Autodesk Inventor part; units mm, degrees
ref_plane "YZ Plane" through (0, 0, 0) normal (1, 0, 0) x (0, 1, 0)
ref_plane "XZ Plane" through (0, 0, 0) normal (0, 1, 0) x (-1, 0, 0)
ref_plane "XY Plane" through (0, 0, 0) normal (0, 0, 1) x (1, 0, 0)
sketch "Sketch1" plane through (0, 0, 0) normal (0, 1, 0) x (-1, 0, 0)
  circle A0 centre (0, 0) radius 103.75 construction
  line L0 (0, -103.75) -> (-30, -103.75) construction
  line L1 (-30, -103.75) -> (-30, -99.318) construction
  line L2 (0, -103.75) -> (0, -91.6543) construction
  line L3 (0, 0) -> (-10.2863, 0) construction
  circle A1 centre (-30, -99.318) radius 1.6
  circle A2 centre (30, -99.318) radius 1.6
  circle A3 centre (-99.318, -30) radius 1.6
  circle A4 centre (-99.318, 30) radius 1.6
  arc A5 (53.1423, -96.3114) -> (51.7739, -97.0539) centre (0, 0) ccw construction
  arc A6 (43.0581, -98.5) -> (-43.0581, -98.5) centre (0, 0) ccw
  line L4 (0, -107.5) -> (0, -98.5) construction
  line L5 (0, -98.5) -> (0, -73.5) construction
  line L6 (0, -98.5) -> (-43.0581, -98.5) construction
  line L7 (0, -98.5) -> (43.0581, -98.5) construction
  line L8 (43.0581, -98.5) -> (-43.0581, -98.5) construction
  line L9 (-18.0581, -73.5) -> (18.0581, -73.5)
  arc A7 (43.0581, -98.5) -> (18.0581, -73.5) centre (18.0581, -98.5) ccw
  arc A8 (-18.0581, -73.5) -> (-43.0581, -98.5) centre (-18.0581, -98.5) ccw
  line L10 (0, 107.5) -> (0, 97.5) construction
  line L11 (0, 97.5) -> (-22.5, 97.5) construction
  line L12 (-22.5, 97.5) -> (-22.5, 82.5) construction
  line L13 (22.5, 82.5) -> (22.5, 97.5) construction
  line L14 (22.5, 90) -> (-22.5, 90) construction
  line L15 (15, 97.5) -> (-15, 97.5)
  line L16 (-15, 82.5) -> (15, 82.5)
  arc A9 (15, 82.5) -> (15, 97.5) centre (15, 90) ccw
  arc A10 (-15, 97.5) -> (-15, 82.5) centre (-15, 90) ccw
  line L17 (22.5, 82.5) -> (17.5, 82.5) construction
  line L18 (17.5, 82.5) -> (17.5, 77.5) construction
  circle A11 centre (17.5, 77.5) radius 1.6
  circle A12 centre (-17.5, 77.5) radius 1.6
  line L19 (-58.3363, 79.5495) -> (-79.5495, 58.3363)
  arc A13 (-47.7297, 68.9429) -> (-58.3363, 79.5495) centre (-53.033, 74.2462) ccw
  arc A14 (-79.5495, 58.3363) -> (-68.9429, 47.7297) centre (-74.2462, 53.033) ccw
  line L20 (-68.9429, 47.7297) -> (-47.7297, 68.9429)
  circle A15 centre (-67.1751, 42.4264) radius 1.6
  circle A16 centre (-42.4264, 67.1751) radius 1.6
  line L21 (-97.5, 15) -> (-97.5, -15)
  arc A17 (-82.5, 15) -> (-97.5, 15) centre (-90, 15) ccw
  arc A18 (-97.5, -15) -> (-82.5, -15) centre (-90, -15) ccw
  line L22 (-82.5, -15) -> (-82.5, 15)
  circle A19 centre (-77.5, -17.5) radius 1.6
  circle A20 centre (-77.5, 17.5) radius 1.6
  line L23 (-79.5495, -58.3363) -> (-58.3363, -79.5495)
  arc A21 (-68.9429, -47.7297) -> (-79.5495, -58.3363) centre (-74.2462, -53.033) ccw
  arc A22 (-58.3363, -79.5495) -> (-47.7297, -68.9429) centre (-53.033, -74.2462) ccw
  line L24 (-47.7297, -68.9429) -> (-68.9429, -47.7297)
  circle A23 centre (-42.4264, -67.1751) radius 1.6
  circle A24 centre (-67.1751, -42.4264) radius 1.6
  line L25 (-15, -97.5) -> (15, -97.5)
  arc A25 (-15, -82.5) -> (-15, -97.5) centre (-15, -90) ccw
  arc A26 (15, -97.5) -> (15, -82.5) centre (15, -90) ccw
  line L26 (15, -82.5) -> (-15, -82.5)
  circle A27 centre (17.5, -77.5) radius 1.6
  circle A28 centre (-17.5, -77.5) radius 1.6
  line L27 (58.3363, -79.5495) -> (79.5495, -58.3363)
  arc A29 (47.7297, -68.9429) -> (58.3363, -79.5495) centre (53.033, -74.2462) ccw
  arc A30 (79.5495, -58.3363) -> (68.9429, -47.7297) centre (74.2462, -53.033) ccw
  line L28 (68.9429, -47.7297) -> (47.7297, -68.9429)
  circle A31 centre (67.1751, -42.4264) radius 1.6
  circle A32 centre (42.4264, -67.1751) radius 1.6
  line L29 (97.5, -15) -> (97.5, 15)
  arc A33 (82.5, -15) -> (97.5, -15) centre (90, -15) ccw
  arc A34 (97.5, 15) -> (82.5, 15) centre (90, 15) ccw
  line L30 (82.5, 15) -> (82.5, -15)
  circle A35 centre (77.5, 17.5) radius 1.6
  circle A36 centre (77.5, -17.5) radius 1.6
  line L31 (79.5495, 58.3363) -> (58.3363, 79.5495)
  arc A37 (68.9429, 47.7297) -> (79.5495, 58.3363) centre (74.2462, 53.033) ccw
  arc A38 (58.3363, 79.5495) -> (47.7297, 68.9429) centre (53.033, 74.2462) ccw
  line L32 (47.7297, 68.9429) -> (68.9429, 47.7297)
  circle A39 centre (42.4264, 67.1751) radius 1.6
  circle A40 centre (67.1751, 42.4264) radius 1.6
  line L33 (58.3363, -58.3363) -> (51.2652, -51.2652) construction
  line L34 (40.6586, -61.8718) -> (61.8718, -40.6586)
  arc A41 (40.6586, -61.8718) -> (44.5267, -89.5398) centre (53.033, -74.2462) ccw
  arc A42 (89.5398, -44.5267) -> (61.8718, -40.6586) centre (74.2462, -53.033) ccw
  line L35 (0, -73.5) -> (0, -66.5) construction
  arc A43 (44.5267, 89.5398) -> (40.6586, 61.8718) centre (53.033, 74.2462) ccw
  line L36 (61.8718, 40.6586) -> (40.6586, 61.8718)
  arc A44 (61.8718, 40.6586) -> (89.5398, 44.5267) centre (74.2462, 53.033) ccw
  arc A45 (-89.5398, 44.5267) -> (-61.8718, 40.6586) centre (-74.2462, 53.033) ccw
  line L37 (-40.6586, 61.8718) -> (-61.8718, 40.6586)
  arc A46 (-40.6586, 61.8718) -> (-44.5267, 89.5398) centre (-53.033, 74.2462) ccw
  arc A47 (-44.5267, -89.5398) -> (-40.6586, -61.8718) centre (-53.033, -74.2462) ccw
  line L38 (-61.8718, -40.6586) -> (-40.6586, -61.8718)
  arc A48 (-61.8718, -40.6586) -> (-89.5398, -44.5267) centre (-74.2462, -53.033) ccw
  arc A49 (89.5398, -44.5267) -> (89.5398, 44.5267) centre (0, 0) ccw
  arc A50 (-89.5398, 44.5267) -> (-89.5398, -44.5267) centre (0, 0) ccw
  line L39 (43.0581, -98.5) -> (48.0581, -98.5) construction
  line L40 (48.0581, -98.5) -> (48.0581, -88.5) construction
  circle A51 centre (48.0581, -88.5) radius 1.6
  circle A52 centre (-48.0581, -88.5) radius 1.6
  line L41 (18.0581, -66.5) -> (-18.0581, -66.5)
  arc A53 (17.5, -66.5) -> (43.0581, -59.4724) centre (19.5145, -23.8377) ccw
  arc A54 (-44.5267, -58.0038) -> (-18.0581, -66.5) centre (-19.5089, -25.5422) ccw
  circle A55 centre (30, -99.318) radius 1.6
  circle A56 centre (-30, -99.318) radius 1.6
  circle A57 centre (99.318, 30) radius 1.6
  circle A58 centre (99.318, -30) radius 1.6
  line L42 (76.014, -76.014) -> (75.4483, -75.4483) construction
  line L43 (50.8876, -93.7835) -> (51.2652, -94.4888) construction
  line L44 (51.0764, -94.1361) -> (48.0581, -88.5) construction
  line L45 (53.5045, -92.3155) -> (50.7027, -87.0837)
  line L46 (45.4135, -89.9163) -> (48.4318, -95.5524)
  arc A59 (50.7027, -87.0837) -> (45.4135, -89.9163) centre (48.0581, -88.5) ccw
  arc A60 (48.4318, -95.5524) -> (48.6295, -95.8719) centre (51.0764, -94.1361) ccw
  line L47 (102.1437, -30.8474) -> (102.9099, -31.0772) construction
  line L48 (99.318, -30) -> (102.5268, -30.9623) construction
  line L49 (98.4562, -32.8736) -> (101.2359, -33.7072)
  line L50 (103.3886, -28.0888) -> (100.1798, -27.1264)
  arc A61 (100.1798, -27.1264) -> (98.4562, -32.8736) centre (99.318, -30) ccw
  arc A62 (103.7313, -28.2147) -> (103.3886, -28.0888) centre (102.5268, -30.9623) ccw
  arc A63 (53.5045, -92.3155) -> (101.2359, -33.7072) centre (0, 0) ccw
  line L51 (102.1337, 30.8802) -> (102.8973, 31.1189) construction
  line L52 (99.318, 30) -> (102.5155, 30.9996) construction
  line L53 (100.2131, 27.1366) -> (103.4106, 28.1362)
  line L54 (101.2252, 33.7394) -> (98.4229, 32.8634)
  arc A64 (98.4229, 32.8634) -> (100.2131, 27.1366) centre (99.318, 30) ccw
  arc A65 (103.4106, 28.1362) -> (103.721, 28.2524) centre (102.5155, 30.9996) ccw
  arc A66 (102.9706, -27.9634) -> (102.9617, 27.9959) centre (0, 0) ccw
  line L55 (30.9623, 102.5268) -> (30, 99.318) construction
  line L56 (27.1309, 103.6758) -> (26.1686, 100.467)
  line L57 (33.8314, 98.1689) -> (34.6551, 100.9154)
  arc A67 (26.1686, 100.467) -> (33.8314, 98.1689) centre (30, 99.318) ccw
  arc A68 (27.2401, 103.9915) -> (27.1309, 103.6758) centre (30.9623, 102.5268) ccw
  arc A69 (101.2252, 33.7394) -> (34.6551, 100.9154) centre (0, 0) ccw
  arc A70 (44.5267, 89.5398) -> (30.2211, 95.3241) centre (0, 0) ccw
  arc A71 (-33.8314, 98.1689) -> (-26.1686, 100.467) centre (-30, 99.318) ccw
  line L58 (-33.8314, 98.1689) -> (-34.6551, 100.9154)
  line L59 (-27.1309, 103.6758) -> (-26.1686, 100.467)
  arc A72 (-27.1309, 103.6758) -> (-27.2401, 103.9915) centre (-30.9623, 102.5268) ccw
  arc A73 (26.9967, 103.2282) -> (-26.9967, 103.2282) centre (0, 0) ccw
  arc A74 (27.6048, 96.1144) -> (-27.6048, 96.1144) centre (0, 0) ccw
  arc A75 (-30.2211, 95.3241) -> (-44.5267, 89.5398) centre (0, 0) ccw
  line L60 (-101.2252, 33.7394) -> (-98.4229, 32.8634)
  arc A76 (-100.2131, 27.1366) -> (-98.4229, 32.8634) centre (-99.318, 30) ccw
  line L61 (-100.2131, 27.1366) -> (-103.4106, 28.1362)
  arc A77 (-103.721, 28.2524) -> (-103.4106, 28.1362) centre (-102.5155, 30.9996) ccw
  arc A78 (-34.6551, 100.9154) -> (-101.2252, 33.7394) centre (0, 0) ccw
  arc A79 (-102.9617, 27.9959) -> (48.2308, -95.1771) centre (0, 0) ccw
  circle A80 centre (30, 99.318) radius 2
  circle A81 centre (-30, 99.318) radius 2
  line L62 (0, -73.5) -> (0, -72.7)
  line L63 (18.0581, -72.7) -> (-18.0581, -72.7)
  arc A82 (-18.0581, -72.7) -> (-43.8294, -97.2825) centre (-18.0581, -98.5) ccw
  arc A83 (43.8294, -97.2825) -> (-43.8294, -97.2825) centre (0, 0) ccw
  arc A84 (43.8294, -97.2825) -> (18.0581, -72.7) centre (18.0581, -98.5) ccw
  circle A85 centre (-48.0581, -88.5) radius 1.6
  circle A86 centre (-99.318, -30) radius 1.6
  line L64 (-53.5045, -92.3155) -> (-50.7027, -87.0837)
  line L65 (-45.4135, -89.9163) -> (-48.4318, -95.5524)
  arc A87 (-45.4135, -89.9163) -> (-50.7027, -87.0837) centre (-48.0581, -88.5) ccw
  arc A88 (-48.6295, -95.8719) -> (-48.4318, -95.5524) centre (-51.0764, -94.1361) ccw
  line L66 (-98.4562, -32.8736) -> (-101.2359, -33.7072)
  line L67 (-103.3886, -28.0888) -> (-100.1798, -27.1264)
  arc A89 (-98.4562, -32.8736) -> (-100.1798, -27.1264) centre (-99.318, -30) ccw
  point P0 (0, 90)
  point P1 (-45.9619, 70.7107)
  point P2 (-82.5, 17.5)
  point P3 (-70.7107, -45.9619)
  point P4 (-17.5, -82.5)
  point P5 (45.9619, -70.7107)
  point P6 (82.5, -17.5)
  point P7 (70.7107, 45.9619)
  point P8 (35.7159, -76.7698)
  point P9 (49.5673, -91.3181)
  point P10 (100.9224, -30.4812)
  point P11 (100.9168, 30.4998)
  point P12 (30.4812, 100.9224)
  point P13 (-27.2401, 103.9915)
  point P14 (-103.721, 28.2524)
  point P15 (-43.8294, -97.2825)
  point P16 (-102.9706, -27.9634)
  point P17 (-48.2308, -95.1771)
  dimension "d10" = 215
  dimension "d6" = 207.5
  dimension "d7" = 30
  dimension "d8" = 3.2
  dimension "d9" = 220
  dimension "d11" = 9
  dimension "d12" = 25
  dimension "d13" = 10
  dimension "d14" = 22.5
  dimension "d15" = 15
  dimension "d16" = 45
  dimension "d17" = 5
  dimension "d18" = 5
  dimension "d19" = 3.2
  dimension "d20" = 86.1162
  dimension "d21" = 45
  dimension "d22" = 360
  dimension "d23" = 10
  dimension "d24" = 7
  dimension "d25" = 360
  dimension "d26" = 5
  dimension "d27" = 10
  dimension "d28" = 3.2
  dimension "d29" = 180
  dimension "d30" = 0.8
  dimension "d31" = 6
  dimension "d32" = 8
  dimension "d33" = 4
  dimension "d34" = 4
  dimension "d37" = 0.8
extrude "Extrusion1" add sketch "Sketch1" along normal blind 27 contours A7 A79 L46 A60 A6 | A60 L46 A83 A63 L50 A62 A6 | A7 L9 L62 L63 A84 A41 A79 | A62 L50 A66 L53 A65 A6 | A79 A82 A47 L63 L62 L9 A8 | A8 A6 A88 L65 A79 | A65 L53 A83 A69 L56 A68 A6 | L46 A59 L45 A83 | A41 A84 | A68 L56 A73 L59 A72 A6 | A83 L49 A61 L50 | A6 A77 L61 A79 L65 A88 | A79 L64 A87 L65 | A82 A47 | A72 L59 A83 A78 L61 A77 A6 | L53 A64 L54 A83 | A83 L57 A67 L56 | A79 L67 A89 L66 | L59 A71 L58 A83 | A83 L60 A76 L61
fillet "Fillet1" radius 1 18 edges at (-102.9706, 13.5, -27.9634) (-101.2359, 13.5, -33.7072) (-101.2252, 13.5, 33.7394) (-102.9617, 13.5, 27.9959) (-53.5045, 13.5, -92.3155) (-48.2308, 13.5, -95.1771) (53.5045, 13.5, -92.3155) (48.2308, 13.5, -95.1771) (102.9706, 13.5, -27.9634) (101.2359, 13.5, -33.7072) (102.9617, 13.5, 27.9959) (101.2252, 13.5, 33.7394) (-34.6551, 13.5, 100.9154) (34.6551, 13.5, 100.9154) (-43.8294, 13.5, -97.2825) (43.8294, 13.5, -97.2825) (-26.9967, 13.5, 103.2282) (26.9967, 13.5, 103.2282)
properties part number "Schutz4"
Model file for the job. Use its own axes, mm. A direction names the side the tool comes from. Coordinates: 2 decimals unless noted, no trailing zeros. Loops run counter-clockwise (first coordinate to the right, second up) from the corner with the lowest first, then second, coordinate; pieces in that order, holes last. Notation, with made-up numbers: (-36.75, 53) -> (-10.75, 53) arc R23 ccw to (-10.75, 86) -> close; hole circle Ø5 at (64, 77.25). An arc over 180 degrees is marked (long way). Use one line per item in the form item = value. Start each with the question number.
(1) Pull direction X, two halves, no side cores. Call faces 1 (the cylindrical face through (4.11, 13.31, 107.42)), 2 (the cylindrical face through (46.7, 13.311, -85.825)), 3 (the flat face through (40.3, 27, -86.6)): pulls with the +X half, pulls with the -X half, needs draft (parallel to the pull), parting line crosses it, or undercut.
(2) Flat gauge pins, fed straight in: pin 1 (2.5 mm diameter, centred on x = 99.318, z = -30, fed in from -Y); pin 2 (1 mm diameter, centred on y = 19, z = -38, fed in from -X); pin 3 (1.5 mm diameter, centred on y = 14.5, z = -41.5, fed in from +X); pin 4 (12 mm diameter, centred on y = 19, z = 63, fed in from +X). Where does each tip first touch, or does it go through?
(3) Cut at A-A on z = 0. Give the cut face in (x, y).
(4) Cut at D-D on y = 4.75. Give the number of separate pieces and of enclosed holes in the cut face, and give its area (3 significant figures).
(5) Cut at B-B on x = 57. Give the cut face in (y, z).
(6) Cut at C-C on z = -77. Give the cut face in (x, y) (3 decimals).
(7) Tool access for faces 4 (the cylindrical face through (-75.323, 13.311, 75.573)), 5 (the flat face through (0, 13, -73.5)): list every direction of +Z, -Z, +X, -X, +Y, -Y with a clear straight run to the whole face (end or side of a thin tool).
(8) Probe probe 1 along Z at (x, y) = (30, 5.5); probe 2 along Z at (x, y) = (46, 22.75); probe 3 along X at (y, z) = (16, 49). List the from-to ranges inside material, lowest first. Write a range as from..to.
Values:
q1.face_1 = parting line crosses it
q1.face_2 = undercut
q1.face_3 = needs draft
q2.pin_1 = through
q2.pin_2 = -100.75
q2.pin_3 = 99.48
q2.pin_4 = 91.14
q3.outline = (-107.5, 0) -> (-106.7, 0) -> (-106.7, 27) -> (-107.5, 27) -> close; (106.7, 0) -> (107.5, 0) -> (107.5, 27) -> (106.7, 27) -> close
q4.separate_pieces = 1
q4.enclosed_holes = 9
q4.area = 814 mm2
q5.outline = (0, -91.14) -> (27, -91.14) -> (27, -90.2) -> (0, -90.2) -> close; (0, 90.2) -> (27, 90.2) -> (27, 91.14) -> (0, 91.14) -> close
q6.outline = (-75.015, 0) -> (-73.864, 0) -> (-73.864, 27) -> (-75.015, 27) -> close; (-32.32, 0) -> (-30.815, 0) -> (-30.815, 27) -> (-32.32, 27) -> close; (30.815, 0) -> (32.32, 0) -> (32.32, 27) -> (30.815, 27) -> close; (73.864, 0) -> (75.015, 0) -> (75.015, 27) -> (73.864, 27) -> close
q7.face_4 = +Y, -Y
q7.face_5 = -Z, +Y, -Y
q8.probe_1 = -76.54..-75.63, 95.32..97.32, 101.32..103.23
q8.probe_2 = -97.16..-96.28, -91.01..-86.32, 96.28..97.16
q8.probe_3 = -95.68..-94.78, 94.78..95.68
